Part print with two shaded views. Sizes in mm from the minimum x, y, z corner. Coordinates: 2 decimals unless noted, no trailing zeros. Loops run counter-clockwise (first coordinate to the right, second up) from the corner with the lowest first, then second, coordinate; pieces in that order, holes last. Notation, with made-up numbers: (-29.75, 80.5) -> (28.25, 80.5) arc R22 ccw to (28.25, 101.5) -> close; hole circle Ø11 at (63, -19.75). An arc over 180 degrees is marked (long way). Return JSON: item names as keys, results as strings. Group by question number.
(1) Saw through at B-B on z = 40. Write the cut outline in (x, y), then the cut area to 3 significant figures.
(2) Probe L1, parallel to Z at x = 55, y = 5; L2, parallel to X at y = 2.5, z = 54.5; L3, parallel to Z at x = 40, y = 3.75. List the from-to ranges inside material, lowest first.
(3) Flat gauge pins, fed straight in: pin 1 Ø1 at (x, y) = (59, 7) entering from -Z; pin 2 Ø4 at (x, y) = (15, 7.5) entering from +Z; pin 3 Ø1 at (x, y) = (10, 5) entering from +Z; pin 4 Ø4.5 at (x, z) = (55, 25) entering from +Y. Where does each tip first touch, or does it go through?
(4) Saw through at A-A on x = 40. Write the cut outline in (y, z), then the cut area to 3 significant figures.
(5) Saw through at D-D on z = 55. Write the cut outline in (x, y).
(6) Saw through at C-C on y = 7. Write the cut outline in (x, z).
(7) Mould opens along Z. For the marked faces 1, 2 and 3 say: pulls with the +Z half, pulls with the -Z half, needs draft (parallel to the pull), parting line crosses it, or undercut.
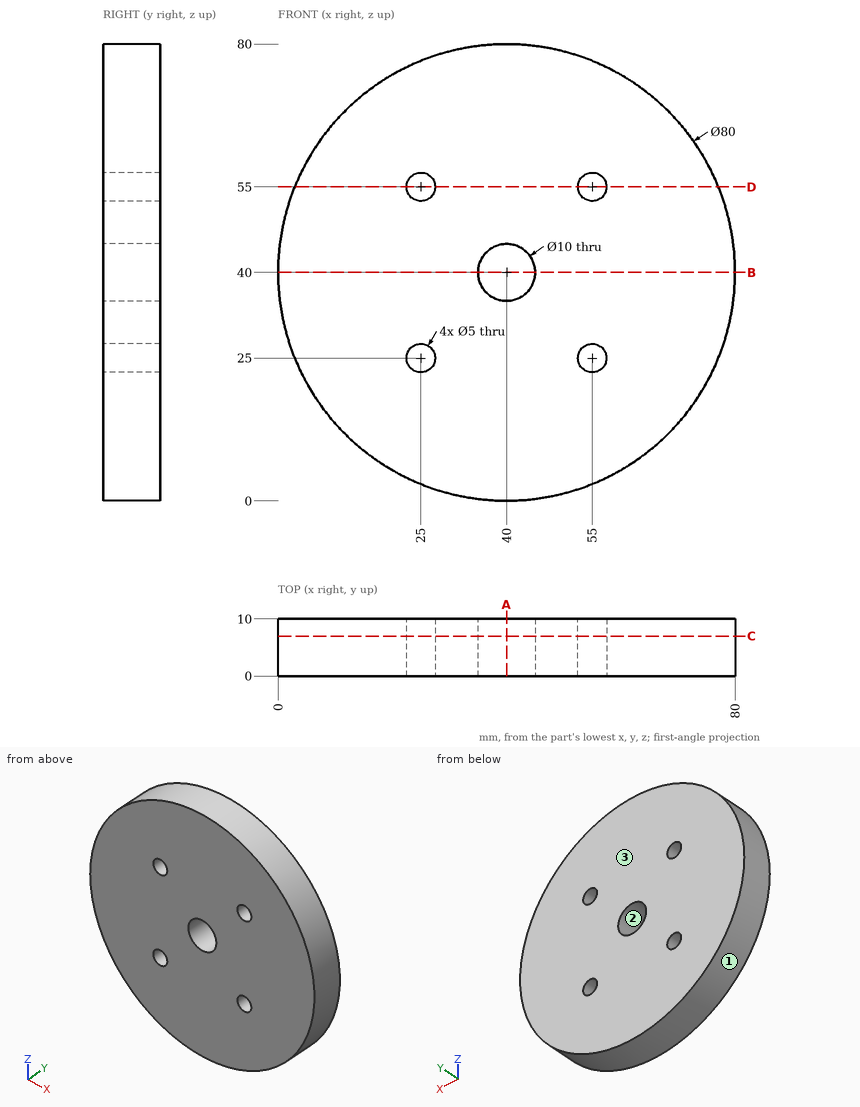
Geometry results:
{
 "1": {"outline": "(0, 0) -> (35, 0) -> (35, 10) -> (0, 10) -> close; (45, 0) -> (80, 0) -> (80, 10) -> (45, 10) -> close", "area": "700 mm²"},
 "2": {"L1": "2.92 to 22.5, 27.5 to 52.5, 57.5 to 77.08", "L2": "2.72 to 22.55, 27.45 to 52.55, 57.45 to 77.28", "L3": "0 to 35, 45 to 80"},
 "3": {"pin 1": "z = 4.54", "pin 2": "z = 72.73", "pin 3": "z = 67.01", "pin 4": "through"},
 "4": {"outline": "(0, 0) -> (10, 0) -> (10, 35) -> (0, 35) -> close; (0, 45) -> (10, 45) -> (10, 80) -> (0, 80) -> close", "area": "700 mm²"},
 "5": {"outline": "(2.92, 0) -> (22.5, 0) -> (22.5, 10) -> (2.92, 10) -> close; (27.5, 0) -> (52.5, 0) -> (52.5, 10) -> (27.5, 10) -> close; (57.5, 0) -> (77.08, 0) -> (77.08, 10) -> (57.5, 10) -> close"},
 "6": {"outline": "circle Ø80 at (40, 40); hole circle Ø5 at (25, 25); hole circle Ø5 at (25, 55); hole circle Ø10 at (40, 40); hole circle Ø5 at (55, 25); hole circle Ø5 at (55, 55)"},
 "7": {"face 1": "parting line crosses it", "face 2": "undercut", "face 3": "needs draft"}
}
